Check sheet for the modelled part. Datum: model origin and axes. Units: mm. Face numbers are marked on the shaded views. A direction names the side the tool comes from. Give positions to 0.01 mm unless a question says otherwise; leave off trailing zeros. Order: outer loops, then holes, each group sorted by start corner. A loop starts at its lowest first (then second) coordinate and runs counter-clockwise, first axis right, second up.
Autodesk Inventor part; units mm, degrees
ref_plane "YZ Plane" through (0, 0, 0) normal (1, 0, 0) x (0, 1, 0)
ref_plane "XZ Plane" through (0, 0, 0) normal (0, 1, 0) x (-1, 0, 0)
ref_plane "XY Plane" through (0, 0, 0) normal (0, 0, 1) x (1, 0, 0)
sketch "Эскиз1" plane through (0, 0, 0) normal (0, 1, 0) x (-1, 0, 0)
  circle A0 centre (0, 0) radius 68
  dimension "d0" = 136
extrude "Выдавливание1" add sketch "Эскиз1" along normal blind 65
sketch "Эскиз2" plane through (0, 0, 0) normal (0, -1, 0) x (1, 0, 0)
  arc A0 (46.7571, -45.1528) -> (64.1997, -10.1682) centre (0, 0) ccw
  line L0 (0, 0) -> (64.1997, -10.1682) construction
  line L1 (0, 0) -> (65, 0) construction
  line L2 (0, 0) -> (46.7571, -45.1528) construction
  arc A1 (-64.1997, -10.1682) -> (-46.7571, -45.1528) centre (0, 0) ccw
  line L3 (0, 0) -> (-64.1997, -10.1682) construction
  line L4 (0, 0) -> (65, 0) construction
  line L5 (0, 0) -> (-46.7571, -45.1528) construction
  line L6 (46.7571, -45.1528) -> (-46.7571, -45.1528)
  line L7 (64.1997, -10.1682) -> (-64.1997, -10.1682)
  dimension "d3" = 65
  dimension "d4" = 9
  dimension "d5" = 35
  dimension "d6" = 65
  dimension "d7" = 171
  dimension "d8" = 35
extrude "Выдавливание2" cut sketch "Эскиз2" against normal blind 65
sketch "Эскиз3" plane through (0, 0, 0) normal (0, -1, 0) x (1, 0, 0)
  arc A0 (64.1997, 10.1682) -> (46.7571, 45.1528) centre (0, 0) ccw
  line L0 (0, 0) -> (64.1997, 10.1682) construction
  line L1 (0, 0) -> (65, 0) construction
  line L2 (0, 0) -> (46.7571, 45.1528) construction
  arc A1 (-46.7571, 45.1528) -> (-64.1997, 10.1682) centre (0, 0) ccw
  line L3 (0, 0) -> (-64.1997, 10.1682) construction
  line L4 (0, 0) -> (65, 0) construction
  line L5 (0, 0) -> (-46.7571, 45.1528) construction
  line L6 (46.7571, 45.1528) -> (-46.7571, 45.1528)
  line L7 (64.1997, 10.1682) -> (-64.1997, 10.1682)
  dimension "d11" = 65
  dimension "d12" = 9
  dimension "d13" = 35
  dimension "d14" = 65
  dimension "d15" = 171
  dimension "d16" = 35
extrude "Выдавливание3" cut sketch "Эскиз3" against normal blind 65
sketch "Эскиз4" plane through (0, 65, 0) normal (0, 1, 0) x (1, 0, 0)
  line L0 (-60, 12.5) -> (60, 12.5)
  line L1 (60, 12.5) -> (60, -12.5)
  line L2 (60, -12.5) -> (-60, -12.5)
  line L3 (-60, -12.5) -> (-60, 12.5)
  line L4 (-60, 12.5) -> (60, -12.5) construction
  line L5 (60, 12.5) -> (-60, -12.5) construction
  point P0 (0, 0)
  dimension "d19" = 120
  dimension "d20" = 25
extrude "Выдавливание4" cut sketch "Эскиз4" against normal blind 62
sketch "Эскиз5" plane through (46.7571, 0, 45.1528) normal (0, 0, -1) x (-1, 0, 0)
  line L0 (89.2571, 15) -> (4.2571, 15)
  line L1 (4.2571, 15) -> (4.2571, 50)
  line L2 (4.2571, 50) -> (89.2571, 50)
  line L3 (89.2571, 50) -> (89.2571, 15)
  line L4 (89.2571, 15) -> (4.2571, 50) construction
  line L5 (4.2571, 15) -> (89.2571, 50) construction
  point P0 (46.7571, 0)
  point P1 (46.7571, 32.5)
  dimension "d23" = 85
  dimension "d24" = 35
extrude "Выдавливание5" cut sketch "Эскиз5" against normal blind 62
chamfer "Фаска1" distance 5 angle 45 1 edges at (0, 15, 45.1528)
chamfer "Фаска2" distance 5 angle 45 1 edges at (0, 50, 68)
fillet "Сопряжение1" radius 10 1 edges at (-60, 3, 0)
fillet "Сопряжение2" radius 10 1 edges at (60, 3, 0)
fillet "Сопряжение3" radius 4 1 edges at (-64.1997, 32.5, 10.1682)
fillet "Сопряжение4" radius 4 1 edges at (-64.1997, 32.5, -10.1682)
fillet "Сопряжение5" radius 4 1 edges at (64.1997, 32.5, -10.1682)
fillet "Сопряжение6" radius 4 1 edges at (64.1997, 32.5, 10.1682)
fillet "Сопряжение7" radius 4 1 edges at (-46.7571, 32.5, -45.1528)
fillet "Сопряжение8" radius 4 1 edges at (46.7571, 32.5, -45.1528)
fillet "Сопряжение9" radius 4 1 edges at (-46.7571, 32.5, 45.1528)
fillet "Сопряжение10" radius 4 1 edges at (46.7571, 32.5, 45.1528)
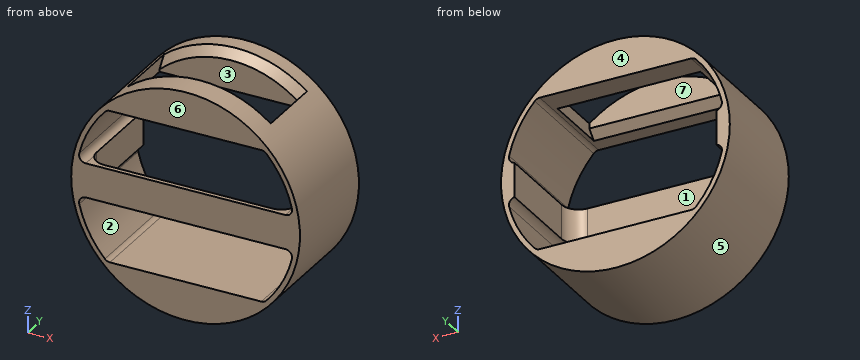
1) Material ranges on L1, parallel to Z at x = 32, y = 6.5; L2, parallel to Z at x = -10, y = 52.5; L3, parallel to X at y = 31.5, z = 38, recorded low to high.
Recorded:
L1: z = -60 to -45.15, 45.15 to 60
L2: z = -67.26 to -45.15, 45.15 to 64.73
L3: x = -56.39 to -52.74, 52.74 to 56.39
2) Section check C-C, the plane x = -52. Record the cut outline in (y, z).
Recorded:
outline: (0, -43.82) - (65, -43.82) - (65, -39) - (0, -39) - close; (0, -10.17) - (3.2, -10.17) - (3.2, 10.17) - (0, 10.17) - close; (0, 39) - (65, 39) - (65, 43.82) - (0, 43.82) - close
3) Section check B-B, the plane z = -41. Record the cut outline in (x, y).
Recorded:
outline: (-54.25, 0) - (-50.44, 0) - (-50.44, 65) - (-54.25, 65) - close; (50.44, 0) - (54.25, 0) - (54.25, 65) - (50.44, 65) - close
4) Depth check by flat-ended pin: pin 1 Ø7.5 at (x, y) = (-22.5, 5.5) entering from -Z; pin 2 Ø10 at (x, z) = (-1, -4) entering from +Y; pin 3 Ø4 at (x, y) = (-32, 26) entering from +Z. Enter the tip coordinate at first touch or a pass-through.
Recorded:
pin 1: stops at z = -65.36
pin 2: stops at y = 3
pin 3: stops at z = -45.15
5) Draft check along X on the marked faces 5, 6 and 7. Enter one of: +X half, -X half, draft (parallel to the pull), parting line (faces both ways), or undercut.
Recorded:
face 5: parting line
face 6: draft
face 7: undercut
6) Section check D-D, the plane z = 0. Record the cut outline in (x, y).
Recorded:
outline: (-68, 0) - (68, 0) - (68, 65) - (60, 65) - (60, 13) arc R10 cw to (50, 3) - (-50, 3) arc R10 cw to (-60, 13) - (-60, 65) - (-68, 65) - close
7) Set-up check for the marked faces 1, 2, 3 and 4: record each of +Z, -Z, +X, -X, +Y, -Y from which the full face is reachable in a straight line by a thin tool's end or side.
Recorded:
face 1: +Y
face 2: +Y, -Y
face 3: +Z
face 4: +Z, -Z, +X, -X, +Y
8) Section check A-A, the plane x = 0. Record the cut outline in (y, z), then the cut area to 3 significant figures.
Recorded:
outline: (0, -68) - (65, -68) - (65, -45.15) - (0, -45.15) - close; (0, -10.17) - (3, -10.17) - (3, 10.17) - (0, 10.17) - close; (0, 45.15) - (10, 45.15) - (15, 50.15) - (15, 68) - (0, 68) - close; (50, 45.15) - (65, 45.15) - (65, 68) - (55, 68) - (50, 63) - close
area: 2,210 mm2
